Source: CAD feature listing. Evaluate the final solid. Frame: model axes, mm. Face numbers are marked on the shaded views. A direction names the side the tool comes from. Coordinates: 2 decimals unless noted, no trailing zeros. Write item = value, one per line. Start each with the question number.
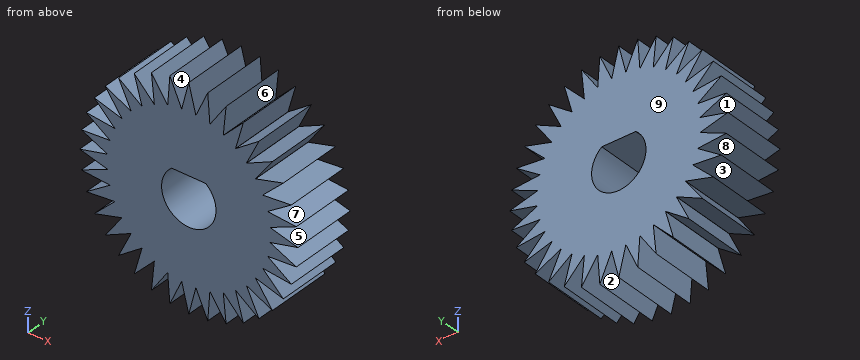
from build123d import *

# Parameters (mm, degrees)
EXTRUDE_2_DEPTH = 6


with BuildPart() as part:
    # Эскиз1 → Бобышка-Вытянуть2 (new body)
    with BuildSketch(Plane(origin=(0, 0, 0), x_dir=(1, 0, 0), z_dir=(0, 1, 0))):
        with BuildLine():
            Line((0, 10.03), (-0.649389435, 7.471833333))
            ThreePointArc((-0.649389435, 7.471833333), (-0.653668071, 7.471460236), (-0.657946491, 7.471084688))
            Line((-0.657946491, 7.471084688), (-1.741691222, 9.877621763))
            Line((-1.741691222, 9.877621763), (-1.936993993, 7.245554104))
            ThreePointArc((-1.936993993, 7.245554104), (-1.941142838, 7.244443697), (-1.945291047, 7.243330915))
            Line((-1.945291047, 7.243330915), (-3.430462038, 9.425116986))
            Line((-3.430462038, 9.425116986), (-3.165743968, 6.799122379))
            ThreePointArc((-3.165743968, 6.799122379), (-3.169636963, 6.797308403), (-3.173528919, 6.795492197))
            Line((-3.173528919, 6.795492197), (-5.015, 8.6862348))
            Line((-5.015, 8.6862348), (-4.298304415, 6.146102762))
            ThreePointArc((-4.298304415, 6.146102762), (-4.301823273, 6.143640332), (-4.30534072, 6.141175888))
            Line((-4.30534072, 6.141175888), (-6.447159725, 7.683425764))
            Line((-6.447159725, 7.683425764), (-5.300263057, 5.306336922))
            ThreePointArc((-5.300263057, 5.306336922), (-5.303300859, 5.303300859), (-5.306336922, 5.300263057))
            Line((-5.306336922, 5.300263057), (-7.683425764, 6.447159725))
            Line((-7.683425764, 6.447159725), (-6.141175888, 4.30534072))
            ThreePointArc((-6.141175888, 4.30534072), (-6.143640332, 4.301823273), (-6.146102762, 4.298304415))
            Line((-6.146102762, 4.298304415), (-8.6862348, 5.015))
            Line((-8.6862348, 5.015), (-6.795492197, 3.173528919))
            ThreePointArc((-6.795492197, 3.173528919), (-6.797308403, 3.169636963), (-6.799122379, 3.165743968))
            Line((-6.799122379, 3.165743968), (-9.425116986, 3.430462038))
            Line((-9.425116986, 3.430462038), (-7.243330915, 1.945291047))
            ThreePointArc((-7.243330915, 1.945291047), (-7.244443697, 1.941142838), (-7.245554104, 1.936993993))
            Line((-7.245554104, 1.936993993), (-9.877621763, 1.741691222))
            Line((-9.877621763, 1.741691222), (-7.471084688, 0.657946491))
            ThreePointArc((-7.471084688, 0.657946491), (-7.471460236, 0.653668071), (-7.471833333, 0.649389435))
            Line((-7.471833333, 0.649389435), (-10.03, 0))
            Line((-10.03, 0), (-7.471833333, -0.649389435))
            ThreePointArc((-7.471833333, -0.649389435), (-7.471460236, -0.653668071), (-7.471084688, -0.657946491))
            Line((-7.471084688, -0.657946491), (-9.877621763, -1.741691222))
            Line((-9.877621763, -1.741691222), (-7.245554104, -1.936993993))
            ThreePointArc((-7.245554104, -1.936993993), (-7.244443697, -1.941142838), (-7.243330915, -1.945291047))
            Line((-7.243330915, -1.945291047), (-9.425116986, -3.430462038))
            Line((-9.425116986, -3.430462038), (-6.799122379, -3.165743968))
            ThreePointArc((-6.799122379, -3.165743968), (-6.797308403, -3.169636963), (-6.795492197, -3.173528919))
            Line((-6.795492197, -3.173528919), (-8.6862348, -5.015))
            Line((-8.6862348, -5.015), (-6.146102762, -4.298304415))
            ThreePointArc((-6.146102762, -4.298304415), (-6.143640332, -4.301823273), (-6.141175888, -4.30534072))
            Line((-6.141175888, -4.30534072), (-7.683425764, -6.447159725))
            Line((-7.683425764, -6.447159725), (-5.306336922, -5.300263057))
            ThreePointArc((-5.306336922, -5.300263057), (-5.303300859, -5.303300859), (-5.300263057, -5.306336922))
            Line((-5.300263057, -5.306336922), (-6.447159725, -7.683425764))
            Line((-6.447159725, -7.683425764), (-4.30534072, -6.141175888))
            ThreePointArc((-4.30534072, -6.141175888), (-4.301823273, -6.143640332), (-4.298304415, -6.146102762))
            Line((-4.298304415, -6.146102762), (-5.015, -8.6862348))
            Line((-5.015, -8.6862348), (-3.173528919, -6.795492197))
            ThreePointArc((-3.173528919, -6.795492197), (-3.169636963, -6.797308403), (-3.165743968, -6.799122379))
            Line((-3.165743968, -6.799122379), (-3.430462038, -9.425116986))
            Line((-3.430462038, -9.425116986), (-1.945291047, -7.243330915))
            ThreePointArc((-1.945291047, -7.243330915), (-1.941142838, -7.244443697), (-1.936993993, -7.245554104))
            Line((-1.936993993, -7.245554104), (-1.741691222, -9.877621763))
            Line((-1.741691222, -9.877621763), (-0.657946491, -7.471084688))
            ThreePointArc((-0.657946491, -7.471084688), (-0.653668071, -7.471460236), (-0.649389435, -7.471833333))
            Line((-0.649389435, -7.471833333), (0, -10.03))
            Line((0, -10.03), (0.649389435, -7.471833333))
            ThreePointArc((0.649389435, -7.471833333), (0.653668071, -7.471460236), (0.657946491, -7.471084688))
            Line((0.657946491, -7.471084688), (1.741691222, -9.877621763))
            Line((1.741691222, -9.877621763), (1.936993993, -7.245554104))
            ThreePointArc((1.936993993, -7.245554104), (1.941142838, -7.244443697), (1.945291047, -7.243330915))
            Line((1.945291047, -7.243330915), (3.430462038, -9.425116986))
            Line((3.430462038, -9.425116986), (3.165743968, -6.799122379))
            ThreePointArc((3.165743968, -6.799122379), (3.169636963, -6.797308403), (3.173528919, -6.795492197))
            Line((3.173528919, -6.795492197), (5.015, -8.6862348))
            Line((5.015, -8.6862348), (4.298304415, -6.146102762))
            ThreePointArc((4.298304415, -6.146102762), (4.301823273, -6.143640332), (4.30534072, -6.141175888))
            Line((4.30534072, -6.141175888), (6.447159725, -7.683425764))
            Line((6.447159725, -7.683425764), (5.300263057, -5.306336922))
            ThreePointArc((5.300263057, -5.306336922), (5.303300859, -5.303300859), (5.306336922, -5.300263057))
            Line((5.306336922, -5.300263057), (7.683425764, -6.447159725))
            Line((7.683425764, -6.447159725), (6.141175888, -4.30534072))
            ThreePointArc((6.141175888, -4.30534072), (6.143640332, -4.301823273), (6.146102762, -4.298304415))
            Line((6.146102762, -4.298304415), (8.6862348, -5.015))
            Line((8.6862348, -5.015), (6.795492197, -3.173528919))
            ThreePointArc((6.795492197, -3.173528919), (6.797308403, -3.169636963), (6.799122379, -3.165743968))
            Line((6.799122379, -3.165743968), (9.425116986, -3.430462038))
            Line((9.425116986, -3.430462038), (7.243330915, -1.945291047))
            ThreePointArc((7.243330915, -1.945291047), (7.244443697, -1.941142838), (7.245554104, -1.936993993))
            Line((7.245554104, -1.936993993), (9.877621763, -1.741691222))
            Line((9.877621763, -1.741691222), (7.471084688, -0.657946491))
            ThreePointArc((7.471084688, -0.657946491), (7.471460236, -0.653668071), (7.471833333, -0.649389435))
            Line((7.471833333, -0.649389435), (10.03, 0))
            Line((10.03, 0), (7.471833333, 0.649389435))
            ThreePointArc((7.471833333, 0.649389435), (7.471460236, 0.653668071), (7.471084688, 0.657946491))
            Line((7.471084688, 0.657946491), (9.877621763, 1.741691222))
            Line((9.877621763, 1.741691222), (7.245554104, 1.936993993))
            ThreePointArc((7.245554104, 1.936993993), (7.244443697, 1.941142838), (7.243330915, 1.945291047))
            Line((7.243330915, 1.945291047), (9.425116986, 3.430462038))
            Line((9.425116986, 3.430462038), (6.799122379, 3.165743968))
            ThreePointArc((6.799122379, 3.165743968), (6.797308403, 3.169636963), (6.795492197, 3.173528919))
            Line((6.795492197, 3.173528919), (8.6862348, 5.015))
            Line((8.6862348, 5.015), (6.146102762, 4.298304415))
            ThreePointArc((6.146102762, 4.298304415), (6.143640332, 4.301823273), (6.141175888, 4.30534072))
            Line((6.141175888, 4.30534072), (7.683425764, 6.447159725))
            Line((7.683425764, 6.447159725), (5.306336922, 5.300263057))
            ThreePointArc((5.306336922, 5.300263057), (5.303300859, 5.303300859), (5.300263057, 5.306336922))
            Line((5.300263057, 5.306336922), (6.447159725, 7.683425764))
            Line((6.447159725, 7.683425764), (4.30534072, 6.141175888))
            ThreePointArc((4.30534072, 6.141175888), (4.301823273, 6.143640332), (4.298304415, 6.146102762))
            Line((4.298304415, 6.146102762), (5.015, 8.6862348))
            Line((5.015, 8.6862348), (3.173528919, 6.795492197))
            ThreePointArc((3.173528919, 6.795492197), (3.169636963, 6.797308403), (3.165743968, 6.799122379))
            Line((3.165743968, 6.799122379), (3.430462038, 9.425116986))
            Line((3.430462038, 9.425116986), (1.945291047, 7.243330915))
            ThreePointArc((1.945291047, 7.243330915), (1.941142838, 7.244443697), (1.936993993, 7.245554104))
            Line((1.936993993, 7.245554104), (1.741691222, 9.877621763))
            Line((1.741691222, 9.877621763), (0.657946491, 7.471084688))
            ThreePointArc((0.657946491, 7.471084688), (0.653668071, 7.471460236), (0.649389435, 7.471833333))
            Line((0.649389435, 7.471833333), (0, 10.03))
        make_face()
        with BuildLine():
            ThreePointArc((-1.564448785, -1.95), (0, 2.5), (1.564448785, -1.95))
            Line((1.564448785, -1.95), (-1.564448785, -1.95))
        make_face(mode=Mode.SUBTRACT)
    extrude(amount=EXTRUDE_2_DEPTH)


solid = part.part
Item 1: First-contact query: pin 1 (2 mm diameter, centred on y = 1, z = -1.5, fed in from +X); pin 2 (2 mm diameter, centred on y = 2, z = 7, fed in from +X). Flat tips, straight axial feed; report the tip coordinate or a pass-through.
Item 2: Reachability of the marked faces 1, 2, 3, 4 and 5 from +Z, -Z, +X, -X, +Y, -Y: full face, straight path, thin tool, end or side. Return the list, or none.
Item 3: Material intervals for L1, parallel to X at y = 4.4, z = -8.75; L2, parallel to X at y = 2.2, z = 5.5; L3, parallel to X at y = 2.95, z = 1.5, sorted ascending. Write a range as [from, to].
Item 4: Draft query along X for the marked faces 6, 7, 8 and 9. Return one class per face: released by +X, released by -X, zero draft, split by the parting line, or undercut.
Responses:
q1.pin_1 = 9.88
q1.pin_2 = 7.68
q2.face_1 = -X, +Y, -Y
q2.face_2 = -Z, +Y, -Y
q2.face_3 = +Y, -Y
q2.face_4 = +Z, +Y, -Y
q2.face_5 = +X, +Y, -Y
q3.L1 = [-3.36, -2.97], [-1.83, -1.23], [-0.32, 0.32], [1.23, 1.83], [2.97, 3.36]
q3.L2 = [-7, -5.72], [-5.39, 5.39], [5.72, 7]
q3.L3 = [-9.34, -2], [2, 9.34]
q4.face_6 = undercut
q4.face_7 = released by +X
q4.face_8 = released by -X
q4.face_9 = zero draft
